Could you check a few things on this model? Use its own coordinates, in mm. Face numbers are marked on the shaded views. A direction names the side the tool comes from. Give positions to 0.01 mm unless a question says otherwise; leave off trailing zeros. Order: outer loops, then holes, each group sorted by start corner. A loop starts at its lowest first (then second) coordinate and runs counter-clockwise, first axis right, second up. Notation, with made-up numbers: (46.5, 7) -> (92.5, 7) arc R25 cw to (92.5, 38) -> close; hole circle Ø3 at (34, -31). An arc over 180 degrees is marked (long way). Answer as CSV lines item,"result". Start each with the question number.
(1) I need wall thicknesses on L1, parallel to X at y = -2.5, z = 14.5; L2, parallel to X at y = -28.6, z = 13.5; L3, parallel to X at y = -28.7, z = 13.5. Which ranges of each line are inside material? Lowest first, please.
(2) We'd pull the mould along Z, two halves only. Please class the marked faces 1, 2 and 3: released by +Z, released by -Z, zero draft, split by the parting line, or undercut.
(3) I want a section at C-C (y = 3). Please give me the cut outline in (x, z), plus the area to 3 significant figures.
(4) Will these pins go through, and if not, where does the flat tip stop? pin 1 Ø3 at (y, z) = (-19.5, 3) entering from +X; pin 2 Ø3.5 at (x, z) = (10.5, 1) entering from +Y; pin 3 Ø1 at (x, y) = (-6, -16.5) entering from -Z; pin 4 Ø2.5 at (x, z) = (-1.5, 1.5) entering from +Y.
(5) On a 3-axis mill with a long thin cutter (end or side, diameter ignored), from which of +Z, -Z, +X, -X, +Y, -Y can I reach the whole of each face in a straight line? I mean the marked faces 4, 5, 6 and 7. Say none if no direction works.
(6) I want a section at B-B (x = -1.75). Please give me the cut outline in (y, z).
(7) I want a section at D-D (y = 9.5). Please give me the cut outline in (x, z), plus the area to 3 significant figures.
(8) I want a section at A-A (z = 13.5). Please give me the cut outline in (x, y).
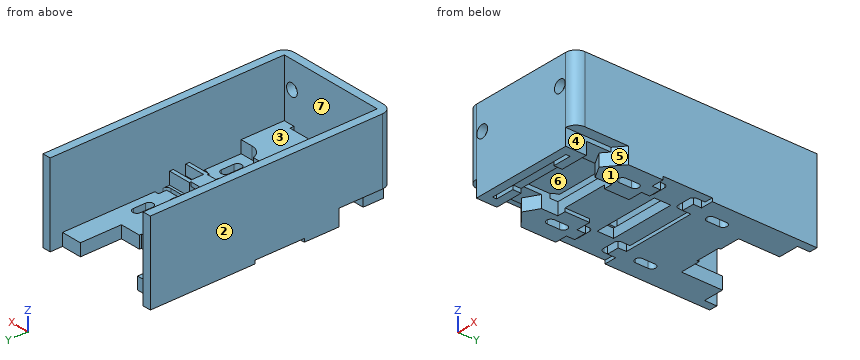
```python
from build123d import *

# Parameters (mm, degrees)
BOSS_EXTRUDE1_DEPTH = 20
CUT_EXTRUDE1_DEPTH  = 39.668462602
CUT_EXTRUDE2_DEPTH  = 39.668462602
SKETCH4_W           = 26
SKETCH4_H           = 57
CUT_EXTRUDE3_DEPTH  = 14
CUT_EXTRUDE4_DEPTH  = 0.8
CUT_EXTRUDE5_DEPTH  = 39.260815464
CUT_EXTRUDE6_DEPTH  = 4
SKETCH8_W           = 5
SKETCH8_H           = 6.5
BOSS_EXTRUDE2_DEPTH = 1
SKETCH9_W           = 20.5
SKETCH9_H           = 1
CUT_EXTRUDE7_DEPTH  = 39.668462602
SKETCH10_W          = 11.5
SKETCH10_H          = 2
CUT_EXTRUDE8_DEPTH  = 1
CUT_EXTRUDE9_DEPTH  = 3
CUT_EXTRUDE10_REACH = 40.668
SKETCH12_W          = 15
SKETCH12_H          = 2
SKETCH13_W          = 16
SKETCH13_H          = 4
CUT_EXTRUDE11_DEPTH = 2.2
SKETCH14_W          = 5
SKETCH14_H          = 3
CUT_EXTRUDE12_DEPTH = 2.5
CUT_EXTRUDE13_REACH = 66.078
SKETCH15_R          = 1.5


with BuildPart() as part:
    # Sketch1 → Boss-Extrude1 (new body)
    with BuildSketch(Plane.XY):
        with BuildLine():
            Line((-15, 29.5), (15, 29.5))
            Line((15, 29.5), (15, -27))
            ThreePointArc((15, -27), (14.267766953, -28.767766953), (12.5, -29.5))
            Line((12.5, -29.5), (-12.5, -29.5))
            ThreePointArc((-12.5, -29.5), (-14.267766953, -28.767766953), (-15, -27))
            Line((-15, -27), (-15, 29.5))
        make_face()
    extrude(amount=BOSS_EXTRUDE1_DEPTH)

    # Sketch2 → Cut-Extrude1 (cut, through all)
    with BuildSketch(Plane(origin=(0, 0, 0), x_dir=(-1, 0, 0), z_dir=(0, 0, -1))):
        Polygon((-13, 29.5), (-13, 26.5), (-8, 26.5), (-8, 16.5), (-3, 16.5), (-3, 16), (3, 16), (3, 16.5), (8, 16.5), (8, 26.5), (13, 26.5), (13, 29.5), align=None)
    extrude(amount=-CUT_EXTRUDE1_DEPTH, mode=Mode.SUBTRACT)

    # Sketch3 → Cut-Extrude2 (cut, through all)
    with BuildSketch(Plane(origin=(0, 0, 0), x_dir=(-1, 0, 0), z_dir=(0, 0, -1))):
        with BuildLine():
            Line((-9, 11), (-9, 8))
            ThreePointArc((-9, 8), (-10, 7), (-11, 8))
            Line((-11, 8), (-11, 11))
            ThreePointArc((-11, 11), (-10, 12), (-9, 11))
        make_face()
        with BuildLine():
            Line((9, 8), (9, 11))
            ThreePointArc((9, 11), (10, 12), (11, 11))
            Line((11, 11), (11, 8))
            ThreePointArc((11, 8), (10, 7), (9, 8))
        make_face()
        with BuildLine():
            Line((9, -13.5), (9, -10.5))
            ThreePointArc((9, -10.5), (10, -9.5), (11, -10.5))
            Line((11, -10.5), (11, -13.5))
            ThreePointArc((11, -13.5), (10, -14.5), (9, -13.5))
        make_face()
        with BuildLine():
            Line((-9, -10.5), (-9, -13.5))
            ThreePointArc((-9, -13.5), (-10, -14.5), (-11, -13.5))
            Line((-11, -13.5), (-11, -10.5))
            ThreePointArc((-11, -10.5), (-10, -9.5), (-9, -10.5))
        make_face()
    extrude(amount=-CUT_EXTRUDE2_DEPTH, mode=Mode.SUBTRACT)

    # Sketch4 → Cut-Extrude3 (cut)
    with BuildSketch(Plane.XY.offset(20)):
        with Locations((0, 1)):
            Rectangle(SKETCH4_W, SKETCH4_H)
    extrude(amount=-CUT_EXTRUDE3_DEPTH, mode=Mode.SUBTRACT)

    # Sketch5 → Cut-Extrude4 (cut)
    with BuildSketch(Plane(origin=(0, 0, 0), x_dir=(-1, 0, 0), z_dir=(0, 0, -1))):
        Polygon((-15, 4), (-12, 4), (-12, 2), (-9, 2), (-9, 4), (9, 4), (9, 2), (12, 2), (12, 4), (15, 4), (15, -8), (12, -8), (12, -6), (9, -6), (9, -8), (5.5, -8), (5.5, -14), (-5.5, -14), (-5.5, -8), (-9, -8), (-9, -6), (-12, -6), (-12, -8), (-15, -8), align=None)
    extrude(amount=-CUT_EXTRUDE4_DEPTH, mode=Mode.SUBTRACT)

    # Sketch6 → Cut-Extrude5 (cut, through all)
    with BuildSketch(Plane(origin=(0, 0, 0.8), x_dir=(-1, 0, 0), z_dir=(0, 0, -1))):
        with BuildLine():
            Line((-12, 4), (-12, 2))
            Line((-12, 2), (-9, 2))
            Line((-9, 2), (-9, 4))
            Line((-9, 4), (-8, 4))
            Line((-8, 4), (-8, 2))
            ThreePointArc((-8, 2), (-8.292893219, 1.292893219), (-9, 1))
            Line((-9, 1), (-12, 1))
            ThreePointArc((-12, 1), (-12.707106781, 1.292893219), (-13, 2))
            Line((-13, 2), (-13, 4))
            Line((-13, 4), (-12, 4))
        make_face()
        with BuildLine():
            Line((13, 4), (12, 4))
            Line((12, 4), (12, 2))
            Line((12, 2), (9, 2))
            Line((9, 2), (9, 4))
            Line((9, 4), (8, 4))
            Line((8, 4), (8, 2))
            ThreePointArc((8, 2), (8.292893219, 1.292893219), (9, 1))
            Line((9, 1), (12, 1))
            ThreePointArc((12, 1), (12.707106781, 1.292893219), (13, 2))
            Line((13, 2), (13, 4))
        make_face()
        with BuildLine():
            Line((12, -8), (12, -6))
            Line((12, -6), (9, -6))
            Line((9, -6), (9, -8))
            Line((9, -8), (8, -8))
            Line((8, -8), (8, -6))
            ThreePointArc((8, -6), (8.292893219, -5.292893219), (9, -5))
            Line((9, -5), (12, -5))
            ThreePointArc((12, -5), (12.707106781, -5.292893219), (13, -6))
            Line((13, -6), (13, -8))
            Line((13, -8), (12, -8))
        make_face()
        with BuildLine():
            Line((-13, -8), (-12, -8))
            Line((-12, -8), (-12, -6))
            Line((-12, -6), (-9, -6))
            Line((-9, -6), (-9, -8))
            Line((-9, -8), (-8, -8))
            Line((-8, -8), (-8, -6))
            ThreePointArc((-8, -6), (-8.292893219, -5.292893219), (-9, -5))
            Line((-9, -5), (-12, -5))
            ThreePointArc((-12, -5), (-12.707106781, -5.292893219), (-13, -6))
            Line((-13, -6), (-13, -8))
        make_face()
    extrude(amount=-CUT_EXTRUDE5_DEPTH, mode=Mode.SUBTRACT)

    # Sketch7 → Cut-Extrude6 (cut)
    with BuildSketch(Plane(origin=(0, 0, 0), x_dir=(-1, 0, 0), z_dir=(0, 0, -1))):
        with BuildLine():
            Line((-7.5, -14), (7.5, -14))
            Line((7.5, -14), (7.5, -18))
            Line((7.5, -18), (10.828862426, -19.921919618))
            Line((10.828862426, -19.921919618), (15, -16.421919618))
            Line((15, -16.421919618), (15, -27))
            ThreePointArc((15, -27), (14.267766953, -28.767766953), (12.5, -29.5))
            Line((12.5, -29.5), (12.5, -24.5))
            Line((12.5, -24.5), (-12.5, -24.5))
            Line((-12.5, -24.5), (-12.5, -29.5))
            ThreePointArc((-12.5, -29.5), (-14.267766953, -28.767766953), (-15, -27))
            Line((-15, -27), (-15, -16.421919618))
            Line((-15, -16.421919618), (-10.828862426, -19.921919618))
            Line((-10.828862426, -19.921919618), (-7.5, -18))
            Line((-7.5, -18), (-7.5, -14))
        make_face()
    extrude(amount=-CUT_EXTRUDE6_DEPTH, mode=Mode.SUBTRACT)

    # Sketch8 → Boss-Extrude2 (add)
    with BuildSketch(Plane(origin=(0, 0, 4), x_dir=(-1, 0, 0), z_dir=(0, 0, -1))):
        with Locations((-10, -21.25)):
            Rectangle(SKETCH8_W, SKETCH8_H)
        with Locations((10, -21.25)):
            Rectangle(SKETCH8_W, SKETCH8_H)
    extrude(amount=BOSS_EXTRUDE2_DEPTH)

    # Sketch9 → Cut-Extrude7 (cut, through all)
    with BuildSketch(Plane(origin=(0, 0, 0), x_dir=(-1, 0, 0), z_dir=(0, 0, -1))):
        with Locations((0, -27)):
            Rectangle(SKETCH9_W, SKETCH9_H)
    extrude(amount=-CUT_EXTRUDE7_DEPTH, mode=Mode.SUBTRACT)

    # Sketch10 → Cut-Extrude8 (cut)
    with BuildSketch(Plane(origin=(0, 0, 0), x_dir=(-1, 0, 0), z_dir=(0, 0, -1))):
        with Locations((0, -25.5)):
            Rectangle(SKETCH10_W, SKETCH10_H)
    extrude(amount=-CUT_EXTRUDE8_DEPTH, mode=Mode.SUBTRACT)

    # Sketch11 → Cut-Extrude9 (cut)
    with BuildSketch(Plane.XY.offset(6)):
        Polygon((-13, 26.5), (-13, 0.4), (-7.5, 0.4), (-7.5, 0), (7.5, 0), (7.5, 0.4), (13, 0.4), (13, 26.5), align=None)
        with BuildLine():
            Line((7.5, -4.4), (13, -4.4))
            Line((13, -4.4), (13, -17))
            Line((13, -17), (10, -17))
            ThreePointArc((10, -17), (7.869334998, -16.276736691), (6.619259608, -14.405866658))
            Line((6.619259608, -14.405866658), (-6.619259608, -14.405866658))
            ThreePointArc((-6.619259608, -14.405866658), (-7.869334998, -16.276736691), (-10, -17))
            Line((-10, -17), (-13, -17))
            Line((-13, -17), (-13, -4.4))
            Line((-13, -4.4), (-7.5, -4.4))
            Line((-7.5, -4.4), (-7.5, -4))
            Line((-7.5, -4), (7.5, -4))
            Line((7.5, -4), (7.5, -4.4))
        make_face()
    extrude(amount=-CUT_EXTRUDE9_DEPTH, mode=Mode.SUBTRACT)

    # Sketch12 → Cut-Extrude10 (cut, up to next)
    with BuildSketch(Plane(origin=(0, 0, 0), x_dir=(1, 0, 0), z_dir=(0, 1, 0)), mode=Mode.PRIVATE) as cut_extrude10_sk1:
        with Locations((0, -4)):
            Rectangle(SKETCH12_W, SKETCH12_H)
    cut_extrude10_tool1 = extrude(cut_extrude10_sk1.sketch, amount=-CUT_EXTRUDE10_REACH, mode=Mode.PRIVATE) & part.part
    add(cut_extrude10_tool1.solids().sort_by_distance((0, 0, 4))[0], mode=Mode.SUBTRACT)

    # Sketch13 → Cut-Extrude11 (cut)
    with BuildSketch(Plane(origin=(0, 0, 0.8), x_dir=(-1, 0, 0), z_dir=(0, 0, -1))):
        with Locations((0, -2)):
            Rectangle(SKETCH13_W, SKETCH13_H)
    extrude(amount=-CUT_EXTRUDE11_DEPTH, mode=Mode.SUBTRACT)

    # Sketch14 → Cut-Extrude12 (cut)
    with BuildSketch(Plane.XY.offset(6)):
        with Locations((-10.5, -2)):
            Rectangle(SKETCH14_W, SKETCH14_H)
        with Locations((10.5, -2)):
            Rectangle(SKETCH14_W, SKETCH14_H)
    extrude(amount=-CUT_EXTRUDE12_DEPTH, mode=Mode.SUBTRACT)

    # Sketch15 → Cut-Extrude13 (cut, up to next)
    with BuildSketch(Plane.XZ.offset(29.5), mode=Mode.PRIVATE) as cut_extrude13_sk1:
        with Locations(Location((-10.85, 13.5, 0), (0, 0, 270))):
            Circle(SKETCH15_R)
    cut_extrude13_tool1 = extrude(cut_extrude13_sk1.sketch, amount=-CUT_EXTRUDE13_REACH, mode=Mode.PRIVATE) & part.part
    # Sketch15 → Cut-Extrude13 (cut, up to next)
    with BuildSketch(Plane.XZ.offset(29.5), mode=Mode.PRIVATE) as cut_extrude13_sk2:
        with Locations(Location((10.85, 13.5, 0), (0, 0, 270))):
            Circle(SKETCH15_R)
    cut_extrude13_tool2 = extrude(cut_extrude13_sk2.sketch, amount=-CUT_EXTRUDE13_REACH, mode=Mode.PRIVATE) & part.part
    add(cut_extrude13_tool1.solids().sort_by_distance((-10.85, -29.5, 13.5))[0], mode=Mode.SUBTRACT)
    add(cut_extrude13_tool2.solids().sort_by_distance((10.85, -29.5, 13.5))[0], mode=Mode.SUBTRACT)


solid = part.part
```
Final values:
1,L1,"-15 to -13, 13 to 15"
1,L2,"-14.42 to -12.35, -9.35 to 9.35, 12.35 to 14.42"
1,L3,"-14.33 to -12.35, -9.35 to 9.35, 12.35 to 14.33"
2,face 1,"released by -Z"
2,face 2,"zero draft"
2,face 3,"released by +Z"
3,outline,"(-15, 0.8) -> (-13, 0.8) -> (-13, 20) -> (-15, 20) -> close; (-12, 0) -> (-9, 0) -> (-9, 3) -> (-12, 3) -> close; (-8, 0.8) -> (8, 0.8) -> (8, 3) -> (-8, 3) -> close; (9, 0) -> (12, 0) -> (12, 3) -> (9, 3) -> close; (13, 0.8) -> (15, 0.8) -> (15, 20) -> (13, 20) -> close"
3,area,"130 mm²"
4,pin 1,"x = 15"
4,pin 2,"y = 26.5"
4,pin 3,"z = 4"
4,pin 4,"y = 16"
5,face 4,"-Z, +X, -Y"
5,face 5,"-Z, +X"
5,face 6,"-Z, +Y"
5,face 7,"+Z"
6,outline,"(-29.5, 0) -> (-27.5, 0) -> (-27.5, 20) -> (-29.5, 20) -> close; (-26.5, 1) -> (-24.5, 1) -> (-24.5, 4) -> (-14.41, 4) -> (-14.41, 6) -> (-26.5, 6) -> close; (-14, 0.8) -> (-4, 0.8) -> (-4, 3) -> (-14, 3) -> close; (-4, 5) -> (0, 5) -> (0, 6) -> (-4, 6) -> close; (0, 0.8) -> (4, 0.8) -> (4, 0) -> (16, 0) -> (16, 3) -> (0, 3) -> close"
7,outline,"(-15, 0) -> (-11, 0) -> (-11, 3) -> (-13, 3) -> (-13, 20) -> (-15, 20) -> close; (-9, 0) -> (9, 0) -> (9, 3) -> (-9, 3) -> close; (11, 0) -> (15, 0) -> (15, 20) -> (13, 20) -> (13, 3) -> (11, 3) -> close"
7,area,"146 mm²"
8,outline,"(-15, -27) arc R2.5 ccw to (-12.5, -29.5) -> (-12.35, -29.5) -> (-12.35, -27.5) -> (-13, -27.5) -> (-13, 29.5) -> (-15, 29.5) -> close; (-9.35, -29.5) -> (9.35, -29.5) -> (9.35, -27.5) -> (-9.35, -27.5) -> close; (12.35, -29.5) -> (12.5, -29.5) arc R2.5 ccw to (15, -27) -> (15, 29.5) -> (13, 29.5) -> (13, -27.5) -> (12.35, -27.5) -> close"
